Check sheet for the modelled part. Datum: model origin and axes. Units: mm. A direction names the side the tool comes from. Round coordinates to 2 decimals unless told otherwise and drop trailing zeros. Order: outer loops, then holes, each group sorted by start corner. A loop starts at its lowest first (then second) coordinate and runs counter-clockwise, first axis right, second up. Notation, with made-up numbers: (71.5, 41) -> (96.5, 41) arc R29 cw to (96.5, 70) -> close; hole circle Ø8 at (16.25, 85). An arc over 180 degrees is marked (long way). Answer in a Markdown table with one row per item.
from build123d import *

# Parameters (mm, degrees)
F1_DEPTH = 25.4
F2_R     = 7.14375
F3_DEPTH = 76.201
F5_DEPTH = 50.8


with BuildPart() as f1:
    # F0 (on Top) → F1 (new body, symmetric)
    with BuildSketch(Plane.XY):
        Polygon((-63.5, 88.9), (-76.2, 88.9), (-76.2, -76.2), (50.8, -76.2), (50.8, -63.5), (-63.5, -63.5), align=None)
    extrude(amount=F1_DEPTH, both=True)

    # F2 (on Right) → F3 (cut, through all)
    with BuildSketch(Plane.YZ):
        with Locations((69.85, 0)):
            Circle(F2_R)
    extrude(amount=-F3_DEPTH, mode=Mode.SUBTRACT)

    # F4 (on face) → F5 (join)
    with BuildSketch(Plane.YZ.offset(50.8)):
        with BuildLine():
            ThreePointArc((-76.2, -2.08e-08), (-69.8499999896, -6.35), (-63.5, 0))
            ThreePointArc((-63.5, 0), (-69.8500000104, 6.35), (-76.2, -2.08e-08))
        make_face()
    extrude(amount=F5_DEPTH)


solid = f1.part
Item 1: Cross-section at A-A (y = 69.85). Record the boundary of the cut face in (x, z), and give its area (3 significant figures).
Result sheet:
| item | result |
|---|---|
| outline | (-76.2, -25.4) -> (-63.5, -25.4) -> (-63.5, -7.14) -> (-76.2, -7.14) -> close; (-76.2, 7.14) -> (-63.5, 7.14) -> (-63.5, 25.4) -> (-76.2, 25.4) -> close |
| area | 464 mm^2 |
Item 2: Cross-section at B-B (z = -15). Record the boundary of the cut face in (x, y), and give its area (3 significant figures).
Result sheet:
| item | result |
|---|---|
| outline | (-76.2, -76.2) -> (50.8, -76.2) -> (50.8, -63.5) -> (-63.5, -63.5) -> (-63.5, 88.9) -> (-76.2, 88.9) -> close |
| area | 3,550 mm^2 |
Item 3: Depth check by flat-ended pin: P1, Ø5, axis at x = 58, z = 7.5, coming from the +Y side; P2, Ø12, axis at y = -30.5, z = -1, coming from the +X side; P3, Ø3, axis at x = 82.5, z = 2, coming from the -Y side. Enter the tip coordinate at first touch or a pass-through.
Result sheet:
| item | result |
|---|---|
| P1 | stops at y = -65.94 |
| P2 | stops at x = -63.5 |
| P3 | stops at y = -76.18 |
Item 4: Cross-section at C-C (y = 49). Record the boundary of the cut face in (x, z), and give its area (3 significant figures).
Result sheet:
| item | result |
|---|---|
| outline | (-76.2, -25.4) -> (-63.5, -25.4) -> (-63.5, 25.4) -> (-76.2, 25.4) -> close |
| area | 645 mm^2 |
Item 5: Mould release check, pull along Z, two halves, no side actions. Record for faces 1 (the cylindrical face through (-69.761, 76.449, -2.736)), 2 (the flat face through (-65, -18, -25.4)), 3 (the flat face through (-63.5, 12, 0)): pulls with the +Z half, pulls with the -Z half, needs draft (parallel to the pull), parting line crosses it, or undercut.
Result sheet:
| item | result |
|---|---|
| face 1 | undercut |
| face 2 | pulls with the -Z half |
| face 3 | needs draft |
Item 6: Set-up check for faces 4 (the flat face through (-6, -63.5, 0)), 5 (the cylindrical face through (75.844, -63.793, 1.907)), 6 (the flat face through (101.6, -70, 0)): record each of +Z, -Z, +X, -X, +Y, -Y from which the full face is reachable in a straight line by a thin tool's end or side.
Result sheet:
| item | result |
|---|---|
| face 4 | +Z, -Z, +X, +Y |
| face 5 | +X |
| face 6 | +Z, -Z, +X, +Y, -Y |
Item 7: Scan lines: line 1 (Z direction, x = -68, y = 69.85); line 2 (X direction, y = -28.5, z = 4). Record each from-to range of solid material in increasing order. Write a range as [from, to].
Result sheet:
| item | result |
|---|---|
| line 1 | z = [-25.4, -7.14], [7.14, 25.4] |
| line 2 | x = [-76.2, -63.5] |
